Geometry: see drawing. Coordinates: mm, zero at the bounding-box minimum. Coordinates: 2 decimals unless noted, no trailing zeros. Loops run counter-clockwise (first coordinate to the right, second up) from the corner with the lowest first, then second, coordinate; pieces in that order, holes last. Notation, with made-up numbers: (89.5, 9.5) - (112.5, 9.5) arc R25 ccw to (112.5, 31.5) - close; hole circle Ø3 at (18, 7.25). An arc over 180 degrees is marked (long way). Use a Markdown table: item, result. Add a question column.
1. Section query B-B on y = 9. Return the cut outline in (x, z).
2. Draft query along Z for the marked faces 1, 2 and 3. Return one class per face: released by +Z, released by -Z, zero draft, split by the parting line, or undercut.
3. Section query A-A on z = 10. Return the cut outline in (x, y), then the cut area to 3 significant figures.
4. Ray query, L1, parallel to Z at x = 27, y = 9; L2, parallel to X at y = 7.5, z = 16.5; L3, parallel to X at y = 8.5, z = 9. Return the intervals inside material, ascending. Write a range as [from, to].
5. Section query C-C on x = 27. Return the cut outline in (y, z), then the cut area to 4 significant figures.
6. Section query D-D on y = 3.75. Return the cut outline in (x, z), then the cut area to 3 significant figures.
7. Contact query for a flat-ended pin moving along its axis: P1, Ø1.5, axis at x = 33, y = 11, coming from the -Z side. Output: stop coordinate, or through.
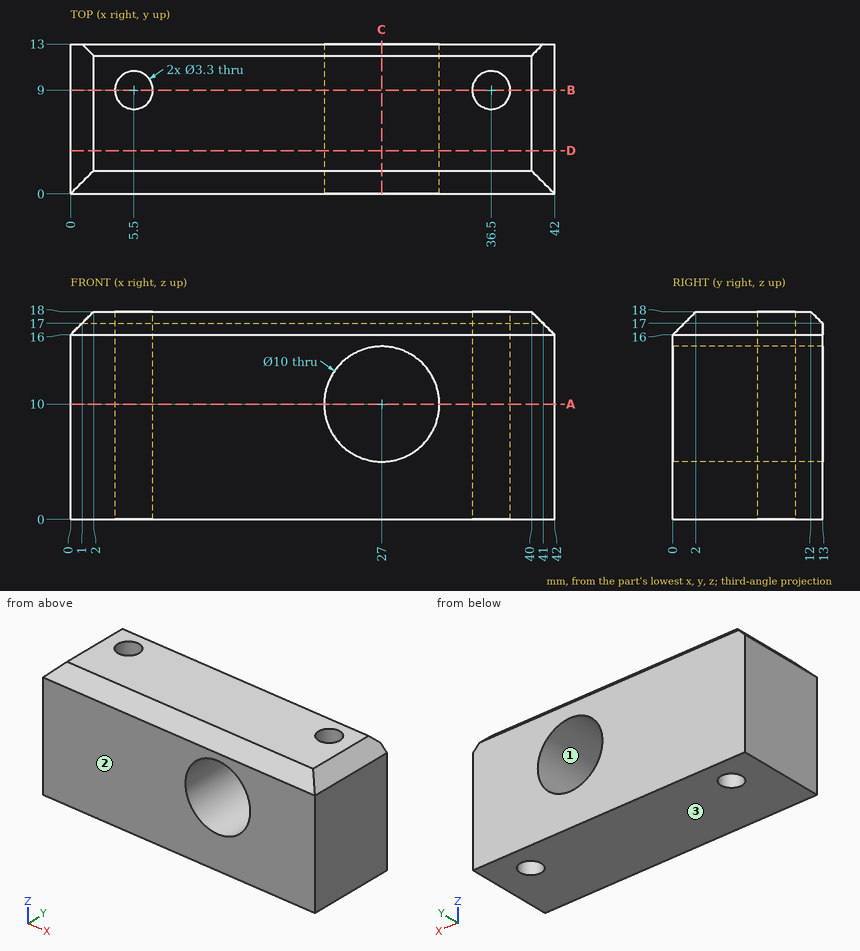
Resolved:
| question | item | result |
|---|---|---|
| 1 | outline | (0, 0) - (3.85, 0) - (3.85, 18) - (2, 18) - (0, 16) - close; (7.15, 0) - (34.85, 0) - (34.85, 18) - (7.15, 18) - close; (38.15, 0) - (42, 0) - (42, 16) - (40, 18) - (38.15, 18) - close; hole circle Ø10 at (27, 10) |
| 2 | face 1 | undercut |
| 2 | face 2 | zero draft |
| 2 | face 3 | released by -Z |
| 3 | outline | (0, 0) - (22, 0) - (22, 13) - (0, 13) - close; (32, 0) - (42, 0) - (42, 13) - (32, 13) - close; hole circle Ø3.3 at (5.5, 9); hole circle Ø3.3 at (36.5, 9) |
| 3 | area | 399 mm² |
| 4 | L1 | [0, 5], [15, 18] |
| 4 | L2 | [0.5, 4.81], [6.19, 35.81], [37.19, 41.5] |
| 4 | L3 | [0, 3.93], [7.07, 22.1], [31.9, 34.93], [38.07, 42] |
| 5 | outline | (0, 0) - (13, 0) - (13, 5) - (0, 5) - close; (0, 15) - (13, 15) - (13, 17) - (12, 18) - (2, 18) - (0, 16) - close |
| 5 | area | 101.5 mm² |
| 6 | outline | (0, 0) - (42, 0) - (42, 16) - (40, 18) - (2, 18) - (0, 16) - close; hole circle Ø10 at (27, 10) |
| 6 | area | 673 mm² |
| 7 | P1 | z = 0 |
